```python
from build123d import *

# Parameters (mm, degrees)
SKETCH_1_R      = 9.5
EXTRUDE_1_DEPTH = 7
EXTRUDE_START   = 7
SKETCH_2_R      = 7
EXTRUDE_2_DEPTH = 6
EXTRUDE_START_2 = 13
SKETCH_3_R      = 9.5
EXTRUDE_3_DEPTH = 7
EXTRUDE_START_3 = 20
SKETCH_4_R      = 12.5
EXTRUDE_4_DEPTH = 10
EXTRUDE_START_4 = 30
SKETCH_5_R      = 10
EXTRUDE_5_DEPTH = 30


with BuildPart() as part:
    # 草图1 → 凸台-拉伸1 (new body)
    with BuildSketch(Plane(origin=(0, 0, 0), x_dir=(1, 0, 0), z_dir=(0, 1, 0))):
        with Locations(Location((0, 0, 0), (0, 0, 270))):
            Circle(SKETCH_1_R)
    extrude(amount=EXTRUDE_1_DEPTH)

    # 草图2 → 凸台-拉伸2 (add)
    with BuildSketch(Plane(origin=(0, 0, 0), x_dir=(1, 0, 0), z_dir=(0, 1, 0)).offset(EXTRUDE_START)):
        with Locations(Location((0, 0, 0), (0, 0, 270))):
            Circle(SKETCH_2_R)
    extrude(amount=EXTRUDE_2_DEPTH)

    # 草图3 → 凸台-拉伸3 (add)
    with BuildSketch(Plane(origin=(0, 0, 0), x_dir=(1, 0, 0), z_dir=(0, 1, 0)).offset(EXTRUDE_START_2)):
        with Locations(Location((0, 0, 0), (0, 0, 270))):
            Circle(SKETCH_3_R)
    extrude(amount=EXTRUDE_3_DEPTH)

    # 草图4 → 凸台-拉伸4 (add)
    with BuildSketch(Plane(origin=(0, 0, 0), x_dir=(1, 0, 0), z_dir=(0, 1, 0)).offset(EXTRUDE_START_3)):
        with Locations(Location((0, 0, 0), (0, 0, 270))):
            Circle(SKETCH_4_R)
    extrude(amount=EXTRUDE_4_DEPTH)

    # 草图5 → 凸台-拉伸5 (add)
    with BuildSketch(Plane(origin=(0, 0, 0), x_dir=(1, 0, 0), z_dir=(0, 1, 0)).offset(EXTRUDE_START_4)):
        with Locations(Location((0, 0, 0), (0, 0, 270))):
            Circle(SKETCH_5_R)
    extrude(amount=EXTRUDE_5_DEPTH)


solid = part.part
```
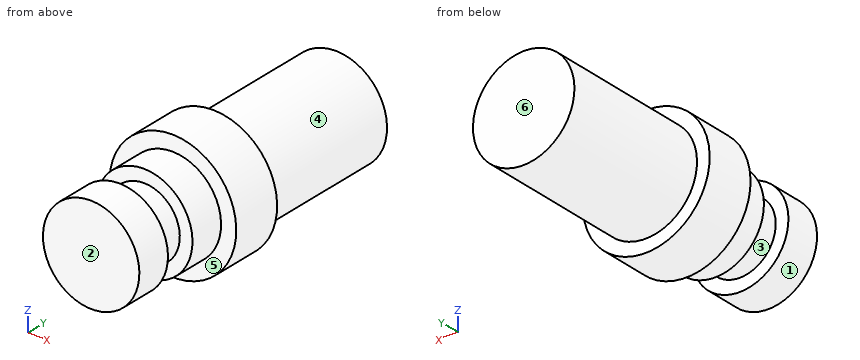
Here's how the part is built. I have some questions about the finished solid (model axes, mm). Face numbers are marked on the shaded views. A direction names the side the tool comes from. Give positions to 0.01 mm unless a question says otherwise; leave off trailing zeros. Write each loop counter-clockwise with the first axis right and the second up, starting at its lowest first coordinate (ties: lowest second). Pieces come first, ordered by that corner, then holes. Notation, with made-up numbers: M 29.25,87.25 L 67.25,87.25 A19 cw 67.25,123.25 Z; hole C 32,26.25 d1. An arc over 180 degrees is marked long. Put each result on its own line as item: value. Start each with the question number.
Item 1: I need wall thicknesses on L1, parallel to Y at x = 3.75, z = 7.5; L2, parallel to X at y = 48, z = 0; L3, parallel to Y at x = 10, z = -7. Which ranges of each line are inside material? Lowest first, please. Write a range as from..to.
Item 2: Will these pins go through, and if not, where does the flat tip stop? pin 1 (6 mm diameter, centred on x = -4, y = 46, fed in from +Z); pin 2 (2 mm diameter, centred on y = 14, z = -4.5, fed in from +X); pin 3 (1 mm diameter, centred on y = 45, z = 6, fed in from +X); pin 4 (12 mm diameter, centred on x = 6.5, z = -1, fed in from -Y).
Item 3: Thinking about a two-plate mould opening in Y: for the marked faces 3, 4, 5 and 6, which applies, +Y half, -Y half, draft (parallel to the pull), parting line (faces both ways), or undercut?
Item 4: On a 3-axis mill with a long thin cutter (end or side, diameter ignored), from which of +Z, -Z, +X, -X, +Y, -Y can I reach the whole of each face in a straight line? I mean the marked faces 1 and 2. Say none if no direction works.
Item 5: If we section it at D-D, the plane y = 27: Write out the boundary of the cut face in (x, z), then the cut area to 3 significant figures.
Item 6: If we section it at B-B, the plane x = 0: Write out the boundary of the cut face in (y, z), then the cut area to 3 significant figures.
Item 7: If we section it at C-C, the plane x = -8.5: Write out the boundary of the cut face in (y, z), then the cut area to 3 significant figures.
Item 8: If we section it at A-A, the plane z = 0: Write out the boundary of the cut face in (x, y).
Values:
1. L1: 0..7, 13..60
1. L2: -10..10
1. L3: 20..30
2. pin 1: z = 9.95
2. pin 2: x = 8.83
2. pin 3: x = 8.35
2. pin 4: y = 0
3. face 3: undercut
3. face 4: draft
3. face 5: -Y half
3. face 6: +Y half
4. face 1: -Y
4. face 2: +Z, -Z, +X, -X, -Y
5. outline: C 0,0 d25
5. area: 491 mm²
6. outline: M 0,-9.5 L 7,-9.5 L 7,-7 L 13,-7 L 13,-9.5 L 20,-9.5 L 20,-12.5 L 30,-12.5 L 30,-10 L 60,-10 L 60,10 L 30,10 L 30,12.5 L 20,12.5 L 20,9.5 L 13,9.5 L 13,7 L 7,7 L 7,9.5 L 0,9.5 Z
6. area: 1,200 mm²
7. outline: M 0,-4.24 L 7,-4.24 L 7,4.24 L 0,4.24 Z; M 13,-4.24 L 20,-4.24 L 20,-9.17 L 30,-9.17 L 30,-5.27 L 60,-5.27 L 60,5.27 L 30,5.27 L 30,9.17 L 20,9.17 L 20,4.24 L 13,4.24 Z
7. area: 618 mm²
8. outline: M -12.5,20 L -9.5,20 L -9.5,13 L -7,13 L -7,7 L -9.5,7 L -9.5,0 L 9.5,0 L 9.5,7 L 7,7 L 7,13 L 9.5,13 L 9.5,20 L 12.5,20 L 12.5,30 L 10,30 L 10,60 L -10,60 L -10,30 L -12.5,30 Z
